from build123d import *

# Parameters (mm, degrees)
SKETCH1_W           = 101.6
SKETCH1_H           = 36.999999914
BOSS_EXTRUDE1_DEPTH = 2.4638
SKETCH2_R           = 5.999999938
SKETCH2_R_2         = 1.750000056
MOTORHOLES_DEPTH    = 55.119869816
SKETCH3_W           = 19.05
SKETCH3_H           = 2.4638
BOTTOMTEETH_DEPTH   = 5.334
SKETCH4_W           = 10.668
SKETCH4_H           = 12.7
CUT_EXTRUDE2_DEPTH  = 57.167338057
SKETCH5_W           = 19.05
SKETCH5_H           = 2.4638
TOPTEETH_DEPTH      = 16.002


with BuildPart() as part:
    # Sketch1 → Boss-Extrude1 (new body)
    with BuildSketch(Plane.XY):
        Rectangle(SKETCH1_W, SKETCH1_H)
    extrude(amount=BOSS_EXTRUDE1_DEPTH)

    # Sketch2 → MotorHoles (cut, through all)
    with BuildSketch(Plane.XY.offset(2.4638)):
        with Locations((0, -8.730000066)):
            Circle(SKETCH2_R)
        with Locations((-10.250000074, -8.730000066)):
            Circle(SKETCH2_R_2)
        with Locations((0, 13.36999993)):
            Circle(SKETCH2_R_2)
        with Locations(Location((10.250000074, -8.730000066, 0), (0, 0, 180))):
            Circle(SKETCH2_R_2)
    extrude(amount=-MOTORHOLES_DEPTH, mode=Mode.SUBTRACT)

    # Sketch3 → BottomTeeth (add)
    with BuildSketch(Plane.XZ.offset(18.499999957)):
        with Locations((-41.275, 1.2319)):
            Rectangle(SKETCH3_W, SKETCH3_H)
        with Locations((41.275, 1.2319)):
            Rectangle(SKETCH3_W, SKETCH3_H)
        with Locations((0, 1.2319)):
            Rectangle(SKETCH3_W, SKETCH3_H)
    extrude(amount=BOTTOMTEETH_DEPTH)

    # Sketch4 → Cut-Extrude2 (cut, through all)
    with BuildSketch(Plane.XY.offset(2.4638)):
        with Locations((-50.8, 0)):
            Rectangle(SKETCH4_W, SKETCH4_H)
        with Locations((50.8, 0)):
            Rectangle(SKETCH4_W, SKETCH4_H)
    extrude(amount=-CUT_EXTRUDE2_DEPTH, mode=Mode.SUBTRACT)

    # Sketch5 → TopTeeth (add)
    with BuildSketch(Plane(origin=(0, 18.499999957, 0), x_dir=(1, 0, 0), z_dir=(0, 1, 0))):
        with Locations((-41.275, -1.2319)):
            Rectangle(SKETCH5_W, SKETCH5_H)
        with Locations((0, -1.2319)):
            Rectangle(SKETCH5_W, SKETCH5_H)
    extrude(amount=TOPTEETH_DEPTH)


solid = part.part
Geometry: final body of the model. Coordinates: model frame, mm. A direction names the side the tool comes from. Round coordinates to 2 decimals unless told otherwise and drop trailing zeros. Loops run counter-clockwise (first coordinate to the right, second up) from the corner with the lowest first, then second, coordinate; pieces in that order, holes last. Notation, with made-up numbers: M -20.5,56 L 35.5,56 A24 cw 35.5,78 Z; hole C -33.75,-11.5 d5. An arc over 180 degrees is marked long. One line per question, with ' | ' between items.
(1) Cut plane D-D on z = 1.25. Give the number of separate pieces and of enclosed holes in the cut face, plus the area to 3 significant figures.
Check result:
separate pieces: 1 | enclosed holes: 4 | area: 4,400 mm2
(2) Cut plane C-C on x = 0. Return the cut outline in (y, z), plus the area to 3 significant figures.
Check result:
outline: M -23.83,0 L -14.73,0 L -14.73,2.46 L -23.83,2.46 Z; M -2.73,0 L 11.62,0 L 11.62,2.46 L -2.73,2.46 Z; M 15.12,0 L 34.5,0 L 34.5,2.46 L 15.12,2.46 Z | area: 106 mm2
(3) Access query for faces 1 (the flat face through (31.75, -21, 1)), 2 (the flat face through (-48, -6.35, 1)), 3 (the flat face through (9.525, 26, 1)). Directions: +Z, -Z, +X, -X, +Y, -Y. A direction counts if a zero-diameter tool reaches every point of the face in a straight line with its end or side. Return the directions, or none.
Check result:
face 1: +Z, -Z, -Y | face 2: +Z, -Z, -X | face 3: +Z, -Z, +X, +Y
(4) Cut plane A-A on y = -8.73. Return the cut outline in (x, z), plus the area to 3 significant figures.
Check result:
outline: M -50.8,0 L -12,0 L -12,2.46 L -50.8,2.46 Z; M -8.5,0 L -6,0 L -6,2.46 L -8.5,2.46 Z; M 6,0 L 8.5,0 L 8.5,2.46 L 6,2.46 Z; M 12,0 L 50.8,0 L 50.8,2.46 L 12,2.46 Z | area: 204 mm2
(5) Material intervals for line 1 along Y through (x, z) = (0, 0.6); line 2 along X through (y, z) = (27.5, 1.3) (3 decimals); line 3 along X through (y, z) = (-8.73, 0.5), sorted ascending. Write a range as from..to.
Check result:
line 1: y = -23.83..-14.73, -2.73..11.62, 15.12..34.5 | line 2: x = -50.8..-31.75, -9.525..9.525 | line 3: x = -50.8..-12, -8.5..-6, 6..8.5, 12..50.8
(6) Contact query for flat-ended pins moving along their axis: P1, Ø0.7, axis at x = 47, z = 1.5, coming from the +Y side; P2, Ø1.2, axis at x = -24.5, z = 1.5, coming from the -Y side. Output: stop coordinate, or through.
Check result:
P1: stops at y = 18.5 | P2: stops at y = -18.5
(7) Cut plane B-B on y = 13.37. Return the cut outline in (x, z), plus the area to 3 significant figures.
Check result:
outline: M -50.8,0 L -1.75,0 L -1.75,2.46 L -50.8,2.46 Z; M 1.75,0 L 50.8,0 L 50.8,2.46 L 1.75,2.46 Z | area: 242 mm2
(8) Pull-direction query (Y, two-part tool) for faces 4 (the cylindrical face through (-9.309, -7.254, 1.249)), 5 (the cylindrical face through (9.3, -10.2, 1.2)), 6 (the flat face through (30, 18.5, 1)), 7 (the flat face through (9.525, -21, 1)); classes: +Y half, -Y half, draft (parallel to the pull), parting line (faces both ways), or undercut.
Check result:
face 4: undercut | face 5: undercut | face 6: +Y half | face 7: draft
